Solid Edge part; units mm, degrees
sketch "Sketch1" plane through (0, 0, 0) normal (0, 0, 1) x (1, 0, 0)
  line L0 (-8, -19.5) -> (8, -19.5)
  line L1 (8, -19.5) -> (8, 19.5)
  line L2 (8, 19.5) -> (-8, 19.5)
  line L3 (-8, 19.5) -> (-8, -19.5)
  circle A0 centre (0, 13) radius 2.6
  circle A1 centre (0, -13) radius 2.6
extrude "Protrusion1" add sketch "Sketch1" along normal blind 8
sketch "Sketch2" plane through (0, 0, 8) normal (0, 0, 1) x (1, 0, 0)
  circle A0 centre (0, 13) radius 4.5
  circle A1 centre (0, -13) radius 4.5
extrude "ExtrudedCutout_1" cut sketch "Sketch2" against normal blind 2
hole "Hole_1" at (-5.5, -19.5, 3) direction (0, 1, 0) diameter 2.459 depth 10 thread major 3 thread length 8
hole "Hole1" at (5.5, -19.5, 3) direction (0, 1, 0) diameter 2.459 depth 10 thread major 3 thread length 8
mirror "Mirror1" about plane through (0, 0, 0) normal (0, 1, 0) of "Hole_1", "Hole1"
Check sheet for the modelled part. Datum: model origin and axes. Units: mm. A direction names the side the tool comes from. Give positions to 0.01 mm unless a question says otherwise; leave off trailing zeros. Order: outer loops, then holes, each group sorted by start corner. A loop starts at its lowest first (then second) coordinate and runs counter-clockwise, first axis right, second up. Notation, with made-up numbers: (8.5, -31.75) -> (53.5, -31.75) arc R27 ccw to (53.5, 4.25) -> close; hole circle Ø9 at (67.25, 17). An arc over 180 degrees is marked (long way). Use CSV: the item, a comma, the result in double quotes. Start each with the question number.
1) Set-up check for faces 1 (the face through (-6, 9.5, 3)), 2 (the face through (-4.41, -14.43, 2.43)), 3 (the face through (-0.56, -10.46, 2.96)), 4 (the face through (2, 11, 6)): record each of +Z, -Z, +X, -X, +Y, -Y from which the full face is reachable in a straight line by a thin tool's end or side.
2) Go/stop test with flat-tipped pins: P1, Ø1.5, axis at x = -5.5, z = 3, coming from the +Y side; P2, Ø5.5, axis at x = 0, y = 13, coming from the -Z side; P3, Ø2.5, axis at x = 0.5, y = -13.5, coming from the +Z side; P4, Ø2, axis at x = 5.5, z = 3, coming from the -Y side. Record where each tip stops, or that it passes through.
3) Sectioned sample at D-D, the plane x = 5.5. Record the boundary of the cut face in (y, z).
4) Sectioned sample at B-B, the plane x = 0. Record the boundary of the cut face in (y, z).
5) Sectioned sample at C-C, the plane z = 7.5. Record the boundary of the cut face in (x, y), plus the area to 3 significant figures.
6) Sectioned sample at A-A, the plane y = -11. Record the boundary of the cut face in (x, z), plus the area to 3 significant figures.
7) Material ranges on line 1 (Y direction, x = 0, z = 3.5); line 2 (X direction, y = -13, z = 3); line 3 (Y direction, x = 0, z = 7.4), recorded low to high. Write a range as from..to.
8) Mould release check, pull along X, two halves, no side actions. Record for faces 5 (the face through (8, 0, 4)), 6 (the face through (0, -19.5, 4)), 7 (the face through (-0.59, -8.54, 7.01)), 8 (the face through (-8, 0, 4)): released by +X, released by -X, zero draft, split by the parting line, or undercut.
Recorded:
1,face 1,"+Y"
1,face 2,"-Y"
1,face 3,"+Z, -Z"
1,face 4,"+Z"
2,P1,"y = 9.5"
2,P2,"z = 0"
2,P3,"through"
2,P4,"y = -9.5"
3,outline,"(-19.5, 0) -> (19.5, 0) -> (19.5, 1.77) -> (9.5, 1.77) -> (9.5, 4.23) -> (19.5, 4.23) -> (19.5, 8) -> (-19.5, 8) -> (-19.5, 4.23) -> (-9.5, 4.23) -> (-9.5, 1.77) -> (-19.5, 1.77) -> close"
4,outline,"(-19.5, 0) -> (-15.6, 0) -> (-15.6, 6) -> (-17.5, 6) -> (-17.5, 8) -> (-19.5, 8) -> close; (-10.4, 0) -> (10.4, 0) -> (10.4, 6) -> (8.5, 6) -> (8.5, 8) -> (-8.5, 8) -> (-8.5, 6) -> (-10.4, 6) -> close; (15.6, 0) -> (19.5, 0) -> (19.5, 8) -> (17.5, 8) -> (17.5, 6) -> (15.6, 6) -> close"
5,outline,"(-8, -19.5) -> (8, -19.5) -> (8, 19.5) -> (-8, 19.5) -> close; hole circle Ø9 at (0, -13); hole circle Ø9 at (0, 13)"
5,area,"497 mm2"
6,outline,"(-8, 0) -> (-1.66, 0) -> (-1.66, 6) -> (-4.03, 6) -> (-4.03, 8) -> (-8, 8) -> close; (1.66, 0) -> (8, 0) -> (8, 8) -> (4.03, 8) -> (4.03, 6) -> (1.66, 6) -> close; hole circle Ø2.46 at (-5.5, 3); hole circle Ø2.46 at (5.5, 3)"
6,area,"82.4 mm2"
7,line 1,"-19.5..-15.6, -10.4..10.4, 15.6..19.5"
7,line 2,"-8..-6.73, -4.27..-2.6, 2.6..4.27, 6.73..8"
7,line 3,"-19.5..-17.5, -8.5..8.5, 17.5..19.5"
8,face 5,"released by +X"
8,face 6,"zero draft"
8,face 7,"undercut"
8,face 8,"released by -X"
